The drawing under review shows one solid part. Ordinate dimensions are in mm from its lowest x, y, z. A direction names the side the tool comes from. Coordinates: 2 decimals unless noted, no trailing zeros. Loops run counter-clockwise (first coordinate to the right, second up) from the corner with the lowest first, then second, coordinate; pieces in that order, holes last. Notation, with made-up numbers: (-32.5, 42.25) - (17.5, 42.25) arc R23 cw to (17.5, 77.25) - close; hole circle Ø11 at (87, 61). An arc over 180 degrees is marked (long way). Answer as a JSON object with one key per item and string values. Group by question number.
Item 1: Mouldability with a two-part tool opening along Y and no side actions: class the marked faces 1, 2 and 3 as released by +Y, released by -Y, zero draft, split by the parting line, or undercut.
Item 2: To check wall thickness, follow line 1 (Z direction, x = 101, y = 64); line 2 (X direction, y = 87.5, z = 10); line 3 (Y direction, x = 102, z = 8.5) (1 decimal). State the ranges of each line that lie inside material, in increasing order.
Item 3: We need section C-C (z = 51.5). Give the boundary of the cut face in (x, y) (1 decimal).
Item 4: Clearance check with flat-ended pins moving along their axes: pin 1 (2 mm diameter, centred on x = 32, z = 18.5, fed in from +Y) (1 decimal); pin 2 (8 mm diameter, centred on y = 83.5, z = 19.5, fed in from +X) (1 decimal); pin 3 (10 mm diameter, centred on x = 111, y = 54, fed in from -Z); pin 4 (1.5 mm diameter, centred on x = 38.5, y = 89, fed in from +Z). State where each tip first meets the part, or that it passes through.
Item 5: Tool access review of the marked faces 4, 5 and 6: name each direction out of +Z, -Z, +X, -X, +Y, -Y from which nothing blocks a thin tool from reaching the whole face with its end or side.
Item 6: We need section A-A (z = 18). Give the boundary of the cut face in (x, y), then the cut area to 3 significant figures.
Item 7: We need section B-B (x = 63.5). Give the boundary of the cut face in (y, z) (1 decimal).
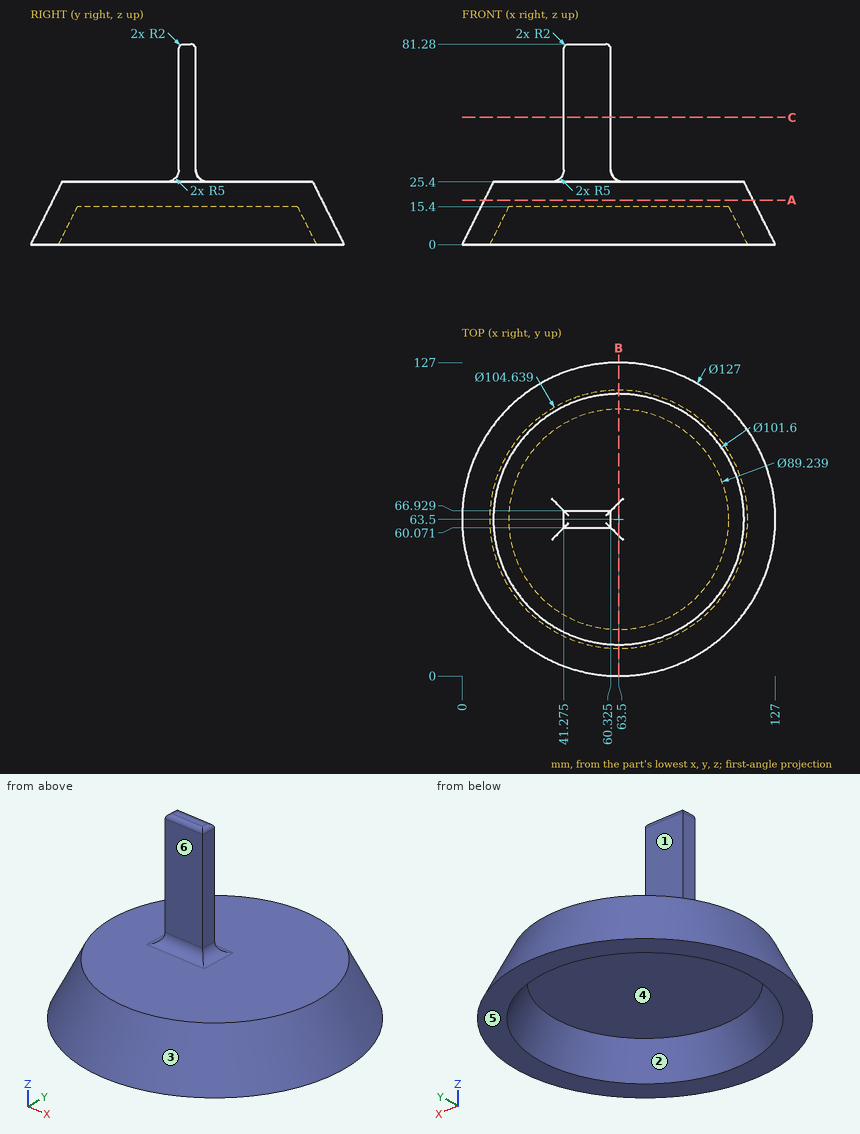
Check sheet entries:
{
 "1": {"face 1": "released by +Y", "face 2": "undercut", "face 3": "split by the parting line"},
 "2": {"line 1": "z = 15.4 to 25.4", "line 2": "x = 10.15 to 22.72, 104.28 to 116.85", "line 3": "y = 18.5 to 34.7, 92.3 to 108.5"},
 "3": {"outline": "(41.3, 60.1) - (60.3, 60.1) - (60.3, 66.9) - (41.3, 66.9) - close"},
 "4": {"pin 1": "stops at y = 108.6", "pin 2": "stops at x = 116", "pin 3": "stops at z = 0", "pin 4": "stops at z = 25.4"},
 "5": {"face 4": "-Z", "face 5": "-Z, +X, -X, +Y, -Y", "face 6": "+Z, +X, -X, -Y"},
 "6": {"outline": "circle Ø109 at (63.5, 63.5)", "area": "9,330 mm2"},
 "7": {"outline": "(0, 0) - (11.2, 0) - (18.9, 15.4) - (108.1, 15.4) - (115.8, 0) - (127, 0) - (114.3, 25.4) - (71.9, 25.4) arc R5 cw to (70.1, 25.7) - (56.9, 25.7) arc R5 cw to (55.1, 25.4) - (12.7, 25.4) - close"}
}
